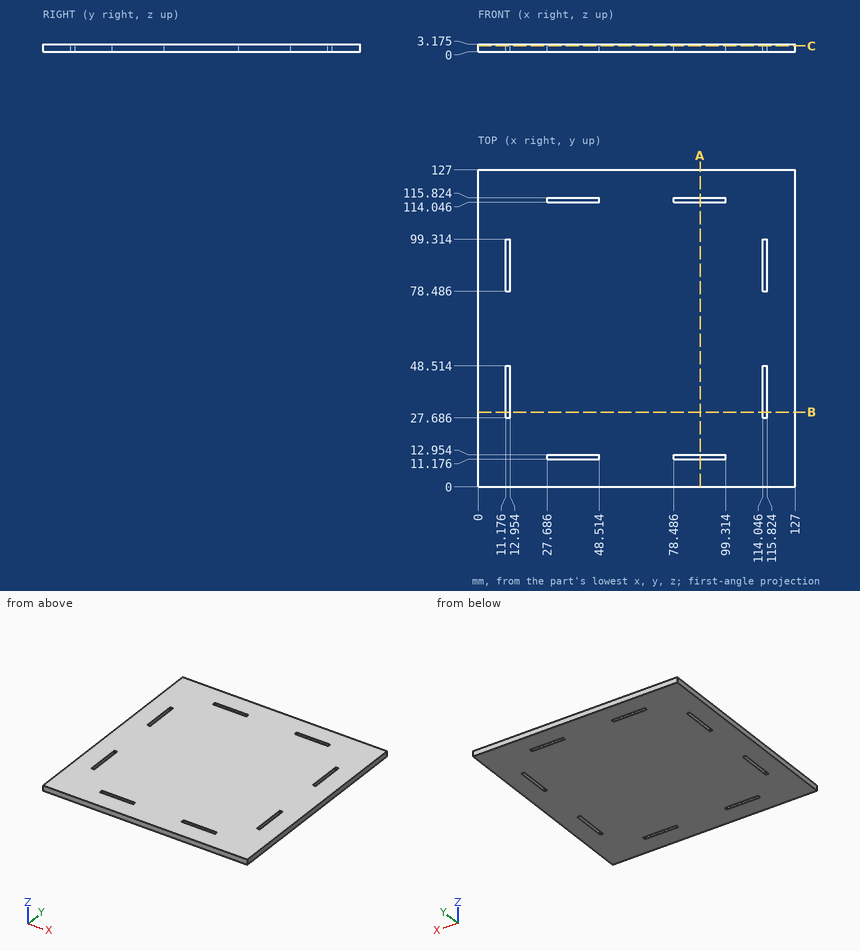
Drawing for the job (mm, zero at the part's lowest x, y, z). Give positions to 0.01 mm unless a question says otherwise; leave off trailing zeros. Loops run counter-clockwise (first coordinate to the right, second up) from the corner with the lowest first, then second, coordinate; pieces in that order, holes last. Notation, with made-up numbers: (-24, 21.5) - (35, 21.5) arc R16 ccw to (35, 45.5) - close; hole circle Ø10 at (0, 10). An arc over 180 degrees is marked (long way). Write item = value, one per line. Start each with the question number.
1) Probe probe 1 along Y at (x, z) = (85.5, 0.15). List the from-to ranges inside material, lowest first. Write a range as from..to.
2) Band-saw the part on A-A on x = 89. Give the cut face in (y, z) (3 decimals), plus the area to 3 significant figures.
3) Band-saw the part on C-C on z = 2.4. Count the separate pieces of the cut face and the enclosed holes in it, plus the area to 3 significant figures.
Final values:
q1.probe_1 = 0..11.18, 12.95..114.05, 115.82..127
q2.outline = (0, 0) - (11.176, 0) - (11.176, 3.175) - (0, 3.175) - close; (12.954, 0) - (114.046, 0) - (114.046, 3.175) - (12.954, 3.175) - close; (115.824, 0) - (127, 0) - (127, 3.175) - (115.824, 3.175) - close
q2.area = 392 mm²
q3.separate_pieces = 1
q3.enclosed_holes = 8
q3.area = 15,800 mm²
